For this review, take the finished solid that the model builds, in its own axes (mm). Face numbers are marked on the shaded views. A direction names the side the tool comes from. Give positions to 0.01 mm unless a question says otherwise; leave off trailing zeros. Write each loop counter-clockwise with the first axis right and the second up, starting at its lowest first coordinate (ties: lowest second). Pieces come first, ordered by that corner, then holes. Notation, with made-up numbers: (55.5, -32) -> (88.5, -32) arc R18 ccw to (88.5, -1) -> close; hole circle Ø8 at (39, 63.5). An arc over 180 degrees is marked (long way). Return JSON: item names as keys, results as strings.
from build123d import *

# Parameters (mm, degrees)
BOSS_EXTRUDE1_START     = -40.32571447
BOSS_EXTRUDE1_DEPTH     = 80.704842411
CUT_EXTRUDE1_DEPTH      = 313.486325482
CUT_EXTRUDE1_DEPTH_BACK = 313.486325482
SKETCH2_W               = 30.352421206
SKETCH2_H               = 220
SKETCH2_W_2             = 30.352421205
SKETCH2_H_2             = 212.373598339
SKETCH5_W               = 79.968077757
SKETCH5_H               = 30.352421206
BOSS_EXTRUDE2_DEPTH     = 7.626401661


# Read off the part's stored shape, not the designer's step: Boss-Extrude1
with BuildPart() as part:
    # Boss-Extrude1 outline → Boss-Extrude1 (new body)
    with BuildSketch(Plane.XY.offset(BOSS_EXTRUDE1_START)):
        Polygon((-31.568063376, 299.369898587), (-31.568063376, 0), (48.400014381, 0), (48.400014381, 292.373598339), align=None)
    extrude(amount=BOSS_EXTRUDE1_DEPTH)

    # Sketch2 → Cut-Extrude1 (cut, two sides: drawn at the far end of the back side and taken through both)
    with BuildSketch(Plane(origin=(48.400014381, 0, 0), x_dir=(0, 0, -1), z_dir=(1, 0, 0)).offset(-CUT_EXTRUDE1_DEPTH_BACK)):
        with Locations((-25.202917338, 150)):
            Rectangle(SKETCH2_W, SKETCH2_H)
        with Locations((25.149503868, 146.18679917)):
            Rectangle(SKETCH2_W_2, SKETCH2_H_2)
    extrude(amount=CUT_EXTRUDE1_DEPTH + CUT_EXTRUDE1_DEPTH_BACK, mode=Mode.SUBTRACT)

    # Sketch5 → Boss-Extrude2 (add)
    with BuildSketch(Plane.XZ.offset(-260)):
        with Locations((8.415975503, 25.202917338)):
            Rectangle(SKETCH5_W, SKETCH5_H)
    extrude(amount=BOSS_EXTRUDE2_DEPTH)


solid = part.part
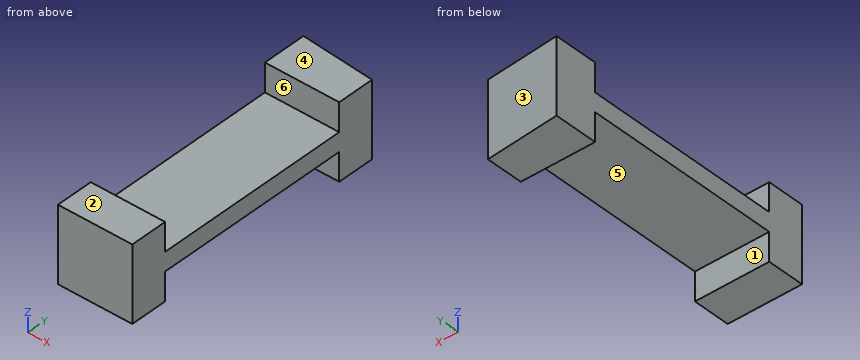
1. Add section B-B, the plane x = -21.5. State the section outline as (y, z) points, plus the area to 3 significant figures.
Results found:
{"outline": "(0, -40.33) -> (40, -40.33) -> (40, -9.97) -> (252.37, -9.97) -> (252.37, -40.33) -> (298.49, -40.33) -> (298.49, 40.38) -> (252.37, 40.38) -> (252.37, 10.03) -> (40, 10.03) -> (40, 40.38) -> (0, 40.38) -> close", "area": "11,200 mm²"}
2. For pin 1 (6 mm diameter, centred on x = -13, z = -10, fed in from -Y); pin 2 (10 mm diameter, centred on x = -12.5, z = -7, fed in from +Y); pin 3 (3 mm diameter, centred on x = -15.5, y = 233.5, fed in from -Z); pin 4 (10 mm diameter, centred on x = -12, y = 149, fed in from +Z), all flat-tipped, find the tip position at first contact; note any pin that passes through.
Results found:
{"pin 1": "stops at y = 0", "pin 2": "stops at y = 298.14", "pin 3": "stops at z = -9.97", "pin 4": "stops at z = 10.03"}
3. For the marked faces 4, 5 and 6, list the 3-axis set-ups (+Z, -Z, +X, -X, +Y, -Y) from which the entire face can be reached by the end or side of a thin tool; tool diameter is ignored.
Results found:
{"face 4": "+Z, +X, -X, +Y, -Y", "face 5": "-Z, +X, -X", "face 6": "+Z, +X, -X"}
4. To check wall thickness, follow probe 1 along Z at (x, y) = (10.5, 242); probe 2 along Y at (x, z) = (-8, -24); probe 3 along Y at (x, z) = (-7, 32). State the ranges of each line that lie inside material, in increasing order.
Results found:
{"probe 1": "z = -9.97 to 10.03", "probe 2": "y = 0 to 40, 252.37 to 297.31", "probe 3": "y = 0 to 40, 252.37 to 297.22"}
5. Add section C-C, the plane y = 236. State the section outline as (x, z) points, plus the area to 3 significant figures.
Results found:
{"outline": "(-31.57, -9.97) -> (48.4, -9.97) -> (48.4, 10.03) -> (-31.57, 10.03) -> close", "area": "1,600 mm²"}
6. Add section A-A, the plane z = -21.5. State the section outline as (x, y) points.
Results found:
{"outline": "(-31.57, 0) -> (48.4, 0) -> (48.4, 40) -> (-31.57, 40) -> close; (-31.57, 252.37) -> (48.4, 252.37) -> (48.4, 292.37) -> (-31.57, 299.37) -> close"}
7. The part is to be moulded in two halves that separate along Y. For the marked faces 1, 2 and 3, say which applies: +Y half, -Y half, draft (parallel to the pull), parting line (faces both ways), or undercut.
Results found:
{"face 1": "undercut", "face 2": "draft", "face 3": "+Y half"}
8. Add section D-D, the plane x = 43.5. State the section outline as (y, z) points.
Results found:
{"outline": "(0, -40.33) -> (40, -40.33) -> (40, -9.97) -> (252.37, -9.97) -> (252.37, -40.33) -> (292.8, -40.33) -> (292.8, 40.38) -> (252.37, 40.38) -> (252.37, 10.03) -> (40, 10.03) -> (40, 40.38) -> (0, 40.38) -> close"}
